Could you check a few things on this drawing? It's one solid part, dimensions in mm from its lowest x, y, z. Round coordinates to 2 decimals unless told otherwise and drop trailing zeros. Write each loop counter-clockwise with the first axis right and the second up, starting at its lowest first coordinate (ties: lowest second). Pieces come first, ordered by that corner, then holes. Notation, with made-up numbers: (13.5, -39.5) - (45.5, -39.5) arc R17 ccw to (45.5, -35.5) - close; hole circle Ø9 at (64.25, 45.25). An arc over 180 degrees is marked (long way). Use one line per item in the form item = value. Start each with the question number.
1. I want a section at A-A, the plane x = 68. List the corners of the cut face in (y, z) for me, plus the area to 3 significant figures.
2. I want a section at B-B, the plane z = 13.75. List the corners of the cut face in (x, y) for me, plus the area to 3 significant figures.
3. We'd pull the mould along Y, two halves only. Please class the marked faces 1, 2, 3 and 4: +Y half, -Y half, draft (parallel to the pull), parting line (faces both ways), or undercut.
4. If I drill on line 1 along Y through (x, z) = (117, 7); line 2 along Y through (x, z) = (68, 5.5); line 3 along Y through (x, z) = (121, 13.5), over which ranges is the centre line in solid material (lowest first)?
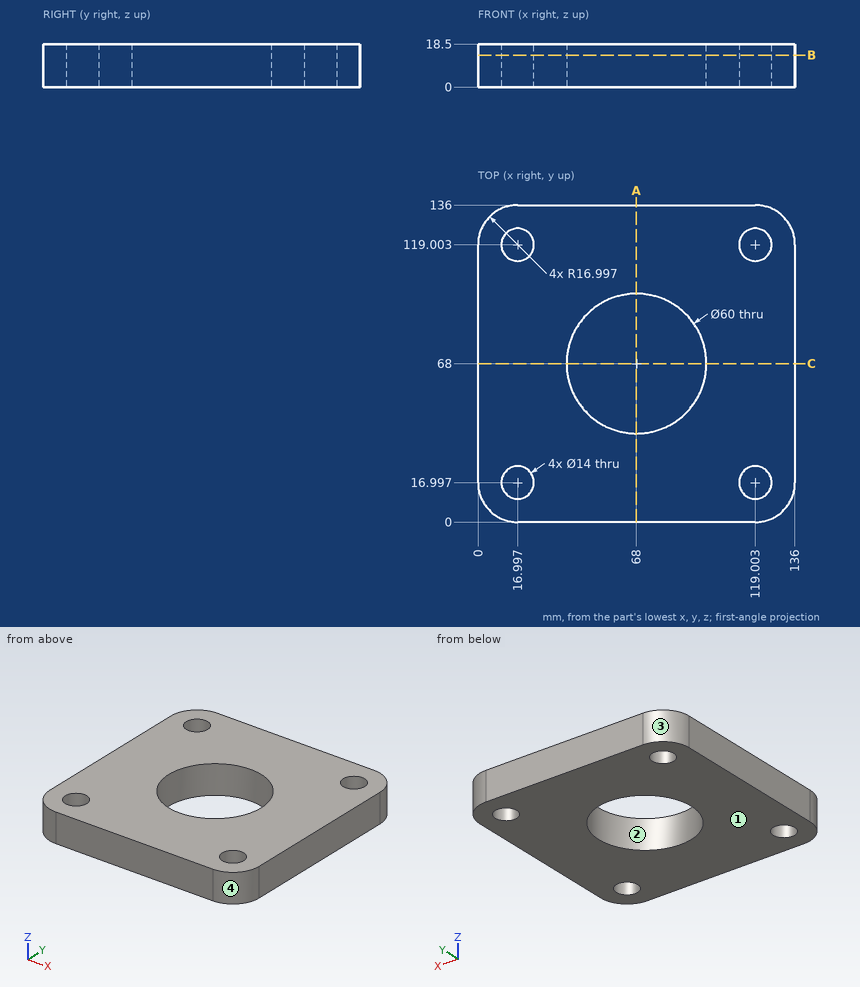
Model answer:
q1.outline = (0, 0) - (38, 0) - (38, 18.5) - (0, 18.5) - close; (98, 0) - (136, 0) - (136, 18.5) - (98, 18.5) - close
q1.area = 1,410 mm2
q2.outline = (0, 17) arc R17 ccw to (17, 0) - (119, 0) arc R17 ccw to (136, 17) - (136, 119) arc R17 ccw to (119, 136) - (17, 136) arc R17 ccw to (0, 119) - close; hole circle Ø14 at (17, 17); hole circle Ø14 at (17, 119); hole circle Ø60 at (68, 68); hole circle Ø14 at (119, 17); hole circle Ø14 at (119, 119)
q2.area = 14,800 mm2
q3.face_1 = draft
q3.face_2 = undercut
q3.face_3 = +Y half
q3.face_4 = -Y half
q4.line_1 = 0 to 10.29, 23.7 to 112.3, 125.71 to 136
q4.line_2 = 0 to 38, 98 to 136
q4.line_3 = 0.12 to 10.29, 23.71 to 112.29, 125.71 to 135.88
